Verification items for the finished model (mm, model axes). Face numbers are marked on the shaded views. A direction names the side the tool comes from. Coordinates: 2 decimals unless noted, no trailing zeros. Order: outer loops, then holes, each group sorted by start corner. A loop starts at its lowest first (then second) coordinate and runs counter-clockwise, first axis right, second up. Notation, with made-up numbers: (53.25, 48) -> (100.25, 48) arc R19 ccw to (100.25, 58) -> close; hole circle Ø6 at (-23, 28.5). An arc over 180 degrees is marked (long way). Write each question's results on one line, items separated by ' | '. Start each with the question number.
(1) Go/stop test with a flat-tipped pin: pin 1 (1 mm diameter, centred on x = 2, z = 2, fed in from -Y). Record where the tip stops, or that it passes through.
(2) Cross-section at A-A on z = 0. Enter the section's corners in (x, y) (3 decimals).
(3) Thickness scan on probe 1 along Z at (x, y) = (0, 3); probe 2 along Y at (x, z) = (2, -1.85); probe 3 along X at (y, z) = (1.25, -0.05). Record the ranges inside material, lowest first. Write a range as [from, to].
(4) Cross-section at C-C on y = 2.25. Enter the section's corners in (x, z), and give its area (3 significant figures).
(5) Cross-section at B-B on x = 0. Enter the section's corners in (y, z) (3 decimals).
(6) Draft check along Z on the marked faces 1, 2 and 3. Enter one of: +Z half, -Z half, draft (parallel to the pull), parting line (faces both ways), or undercut.
(7) Set-up check for the marked faces 4 and 5: record each of +Z, -Z, +X, -X, +Y, -Y from which the full face is reachable in a straight line by a thin tool's end or side.
(8) Cross-section at D-D on z = -1.6. Enter the section's corners in (x, y), and give its area (3 significant figures).
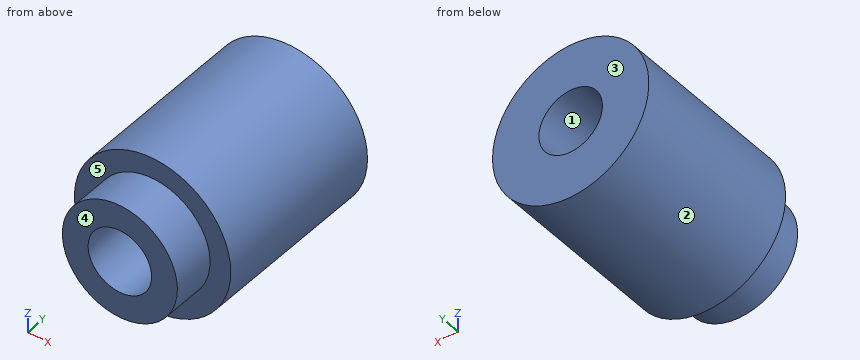
```python
from build123d import *

# Parameters (mm, degrees)
SKETCH1_R             = 2.045
BOSS_EXTRUDE1_DEPTH   = 1.52
SKETCH2_R             = 2.78
BOSS_EXTRUDE2_DEPTH   = 6.35
F_4_40_TAPPED_HOLE1_D = 2.2606


with BuildPart() as part:
    # Sketch1 → Boss-Extrude1 (new body)
    with BuildSketch(Plane(origin=(0, 0, 0), x_dir=(1, 0, 0), z_dir=(0, 1, 0))):
        Circle(SKETCH1_R)
    extrude(amount=BOSS_EXTRUDE1_DEPTH)

    # Sketch2 → Boss-Extrude2 (add)
    with BuildSketch(Plane(origin=(0, 1.52, 0), x_dir=(1, 0, 0), z_dir=(0, 1, 0))):
        Circle(SKETCH2_R)
    extrude(amount=BOSS_EXTRUDE2_DEPTH)

    # #4-40 Tapped Hole1 (through all)
    with Locations(Plane(origin=(0, 7.87, 0), x_dir=(1, 0, 0), z_dir=(0, 1, 0))):
        with Locations((0, 0)):
            Hole(F_4_40_TAPPED_HOLE1_D / 2)


solid = part.part
```
Results are:
1) pin 1: stops at y = 1.52
2) outline: (-2.78, 1.52) -> (-2.045, 1.52) -> (-2.045, 0) -> (-1.13, 0) -> (-1.13, 7.87) -> (-2.78, 7.87) -> close; (1.13, 0) -> (2.045, 0) -> (2.045, 1.52) -> (2.78, 1.52) -> (2.78, 7.87) -> (1.13, 7.87) -> close
3) probe 1: z = [-2.78, -1.13], [1.13, 2.78] | probe 2: y = [1.52, 7.87] | probe 3: x = [-2.04, -1.13], [1.13, 2.04]
4) outline: circle Ø5.56 at (0, 0); hole circle Ø2.26 at (0, 0) | area: 20.3 mm2
5) outline: (0, -2.045) -> (1.52, -2.045) -> (1.52, -2.78) -> (7.87, -2.78) -> (7.87, -1.13) -> (0, -1.13) -> close; (0, 1.13) -> (7.87, 1.13) -> (7.87, 2.78) -> (1.52, 2.78) -> (1.52, 2.045) -> (0, 2.045) -> close
6) face 1: undercut | face 2: parting line | face 3: draft
7) face 4: +Z, -Z, +X, -X, -Y | face 5: -Y
8) outline: (-2.27, 1.52) -> (-1.27, 1.52) -> (-1.27, 0) -> (1.27, 0) -> (1.27, 1.52) -> (2.27, 1.52) -> (2.27, 7.87) -> (-2.27, 7.87) -> close | area: 32.7 mm2
